Read the model definition and answer for the solid it produces. Units are mm, in the model's axes. A direction names the side the tool comes from. Coordinates: 2 decimals unless noted, no trailing zeros. Order: outer loops, then holes, each group sorted by start corner. A loop starts at its lowest first (then second) coordinate and runs counter-clockwise, first axis right, second up. Notation, with made-up numbers: (8, 32.25) -> (37, 32.25) arc R15 cw to (37, 60.25) -> close; hole circle Ø11 at (73.5, 1). An arc over 180 degrees is marked (long way). Use CSV: the item, a comma, the result in double quotes.
```python
from build123d import *

# Parameters (mm, degrees)
BOSS_EXTRUDE1_DEPTH     = 8.36
SKETCH3_R               = 5
BOSS_EXTRUDE2_DEPTH     = 12
CUT_EXTRUDE2_DEPTH      = 22.552948754
CUT_EXTRUDE2_DEPTH_BACK = 22.552948754
CUT_EXTRUDE3_DEPTH      = 22.552948754
CUT_EXTRUDE3_DEPTH_BACK = 22.552948754
SKETCH5_R               = 1.6


with BuildPart() as part:
    # Sketch1 → Boss-Extrude1 (new body)
    with BuildSketch(Plane.XY):
        Polygon((-1.675, 2.901185103), (-3.35, 0), (-1.675, -2.901185103), (1.675, -2.901185103), (3.35, 0), (1.675, 2.901185103), align=None)
    extrude(amount=BOSS_EXTRUDE1_DEPTH)

    # Sketch3 → Boss-Extrude2 (add)
    with BuildSketch(Plane.XY.offset(8.36)):
        Circle(SKETCH3_R)
    extrude(amount=BOSS_EXTRUDE2_DEPTH)

    # Sketch4 → Cut-Extrude2 (cut, two sides: drawn at the far end of the back side and taken through both)
    with BuildSketch(Plane.XY.offset(20.36).offset(-CUT_EXTRUDE2_DEPTH_BACK)):
        with BuildLine():
            Line((-1.565247584, 2.2), (1.565247584, 2.2))
            ThreePointArc((1.565247584, 2.2), (0, -2.7), (-1.565247584, 2.2))
        make_face()
    extrude(amount=CUT_EXTRUDE2_DEPTH + CUT_EXTRUDE2_DEPTH_BACK, mode=Mode.SUBTRACT)

    # Sketch5 → Cut-Extrude3 (cut, two sides: drawn at the far end of the back side and taken through both)
    with BuildSketch(Plane(origin=(0, 0, 0), x_dir=(1, 0, 0), z_dir=(0, 1, 0)).offset(-CUT_EXTRUDE3_DEPTH_BACK)):
        with Locations(Location((0, -14.36, 0), (0, 0, 270))):
            Circle(SKETCH5_R)
    extrude(amount=CUT_EXTRUDE3_DEPTH + CUT_EXTRUDE3_DEPTH_BACK, mode=Mode.SUBTRACT)


solid = part.part
```
Item 1: The mould has two halves that part along Y. Classify faces 1 (the flat face through (-2.5, 1.47, 4.12)), 2 (the flat face through (0, 2.2, 18)), 3 (the flat face through (0, 2.4, 0)), 4 (the flat face through (2.5, -1.47, 4.12)): +Y half, -Y half, draft (parallel to the pull), parting line (faces both ways), or undercut.
Return value:
face 1,"+Y half"
face 2,"undercut"
face 3,"draft"
face 4,"-Y half"
Item 2: Find section D-D, the plane y = 0.5. Give the vertices of the cut face in (x, z), then the cut area to 3 significant figures.
Return value:
outline,"(-4.97, 8.36) -> (-3.06, 8.36) -> (-3.06, 0) -> (-2.65, 0) -> (-2.65, 20.36) -> (-4.97, 20.36) -> close; (2.65, 0) -> (3.06, 0) -> (3.06, 8.36) -> (4.97, 8.36) -> (4.97, 20.36) -> (2.65, 20.36) -> close"
area,"62.5 mm^2"
Item 3: Find section A-A, the plane x = 0. Give the vertices of the cut face in (y, z).
Return value:
outline,"(-5, 8.36) -> (-2.9, 8.36) -> (-2.9, 0) -> (-2.7, 0) -> (-2.7, 12.76) -> (-5, 12.76) -> close; (-5, 15.96) -> (-2.7, 15.96) -> (-2.7, 20.36) -> (-5, 20.36) -> close; (2.2, 0) -> (2.9, 0) -> (2.9, 8.36) -> (5, 8.36) -> (5, 12.76) -> (2.2, 12.76) -> close; (2.2, 15.96) -> (5, 15.96) -> (5, 20.36) -> (2.2, 20.36) -> close"
Item 4: Straight lines are drawn through the part: line 1 along Z through (x, y) = (0, 3.25); line 2 along Z through (x, y) = (-4.5, -1.25); line 3 along Y through (x, z) = (1.75, 11). For each, find the intervals that lie inside material, in ascending order.
Return value:
line 1,"z = 8.36 to 12.76, 15.96 to 20.36"
line 2,"z = 8.36 to 20.36"
line 3,"y = -4.68 to -2.06, 2.06 to 4.68"
Item 5: A tool of negligible diameter and unlimited length cuts with its end or side. For faces 5 (the flat face through (0, 2.901, 4)), 6 (the flat face through (-2.3, -2.2, 8.36)), 7 (the flat face through (2.524, 1.43, 4.121)), from which of +Z, -Z, +X, -X, +Y, -Y can it reach the whole face along a straight path? Write none if from no direction.
Return value:
face 5,"-Z, +X, -X, +Y"
face 6,"-Z"
face 7,"-Z, +X, +Y"
Item 6: Each of these flat-tipped pins is pushed along its axis until it touches: P1, Ø3, axis at x = 2.5, z = 7, coming from the +Y side; P2, Ø3, axis at y = 4, z = 12, coming from the +X side; P3, Ø3.5, axis at x = -0.5, z = 4, coming from the -Y side; P4, Ø3, axis at x = 0, y = 0, coming from the +Z side. Where does it stop, or does it pass through?
Return value:
P1,"stops at y = 4.64"
P2,"stops at x = 4.33"
P3,"stops at y = -2.9"
P4,"passes through"
Item 7: Find section C-C, the plane z = 2. Give the vertices of the cut face in (x, y) (3 decimals), then the cut area to 3 significant figures.
Return value:
outline,"(-3.35, 0) -> (-1.675, -2.901) -> (1.675, -2.901) -> (3.35, 0) -> (1.675, 2.901) -> (-1.675, 2.901) -> close; hole (-1.565, 2.2) arc R2.7 ccw (long way) to (1.565, 2.2) -> close"
area,"7.32 mm^2"
Item 8: Find section B-B, the plane y = 4. Give the vertices of the cut face in (x, z).
Return value:
outline,"(-3, 8.36) -> (3, 8.36) -> (3, 20.36) -> (-3, 20.36) -> close; hole circle Ø3.2 at (0, 14.36)"
